Build history of the part. All positions in model axes, mm. A direction names the side the tool comes from. Give positions to 0.01 mm unless a question says otherwise; leave off trailing zeros. Order: outer loops, then holes, each group sorted by start corner. A loop starts at its lowest first (then second) coordinate and runs counter-clockwise, first axis right, second up. Notation, with made-up numbers: (-29, 32.5) - (-15, 32.5) arc R23 cw to (-15, 44.5) - close; hole circle Ø5 at (55.25, -6). An arc over 180 degrees is marked (long way). Use a Markdown table: item, result.
from build123d import *

# Parameters (mm, degrees)
CUT_EXTRUDE1_DEPTH      = 1.2
CUT_EXTRUDE1_DEPTH_BACK = 1.2


with BuildPart() as part:
    # Sketch1 → Revolve1 (revolve)
    with BuildSketch(Plane.XY):
        with BuildLine():
            Line((-1.782329983, 2.8), (0, 2.8))
            Line((0, 2.8), (0, 1.44675))
            ThreePointArc((0, 1.44675), (0.029289322, 1.376039322), (0.1, 1.34675))
            Line((0.1, 1.34675), (0.428063214, 1.34675))
            Line((0.428063214, 1.34675), (1, 1.5))
            Line((1, 1.5), (8, 1.5))
            Line((8, 1.5), (10, 1.218918331))
            Line((10, 1.218918331), (10, 0))
            Line((10, 0), (-2.4, 0))
            ThreePointArc((-2.4, 0), (-2.267625669, 1.393419223), (-1.875238613, 2.736986301))
            ThreePointArc((-1.875238613, 2.736986301), (-1.838460945, 2.782760589), (-1.782329983, 2.8))
        make_face()
    revolve(axis=Axis((13, 0, 0), (-1, 0, 0)))

    # Sketch2 → Cut-Extrude1 (cut, two sides)
    with BuildSketch(Plane(origin=(-2.4, 0, 0), x_dir=(0, 0, -1), z_dir=(1, 0, 0))) as cut_extrude1_sk:
        Polygon((-1.5, 0.375), (-1.5, -0.375), (-0.6, -0.296260203), (-0.375, -0.375), (-0.296260203, -0.6), (-0.375, -1.5), (0.375, -1.5), (0.296260203, -0.6), (0.375, -0.375), (0.6, -0.296260203), (1.5, -0.375), (1.5, 0.375), (0.6, 0.296260203), (0.375, 0.375), (0.296260203, 0.6), (0.375, 1.5), (-0.375, 1.5), (-0.296260203, 0.6), (-0.375, 0.375), (-0.6, 0.296260203), align=None)
    extrude(amount=CUT_EXTRUDE1_DEPTH, mode=Mode.SUBTRACT)
    extrude(cut_extrude1_sk.sketch, amount=-CUT_EXTRUDE1_DEPTH_BACK, mode=Mode.SUBTRACT)


solid = part.part
1) Wall check: line 1 (Z direction, x = 5.5, y = -0.1); line 2 (Z direction, x = 9, y = -0.2); line 3 (Z direction, x = -1.25, y = -1.3). Give the ranges that are in metal, low to high. Write a range as from..to.
Computed:
| item | result |
|---|---|
| line 1 | z = -1.5..1.5 |
| line 2 | z = -1.34..1.34 |
| line 3 | z = -2.48..-0.36, 0.36..2.48 |
2) Slice it at C-C (x = 3.5). Write the cut outline in (y, z).
Computed:
| item | result |
|---|---|
| outline | circle Ø3 at (0, 0) |
3) Slice it at D-D (x = -0.75). Write the cut outline in (y, z).
Computed:
| item | result |
|---|---|
| outline | circle Ø5.6 at (0, 0) |
4) Tool access for faces 5 (the cylindrical face through (-0.9, -2.8, -0.1)), 6 (the cylindrical face through (4.55, -1.5, -0.07)), 7 (the flat face through (-1.793, -0.336, 1.056)): list every direction of +Z, -Z, +X, -X, +Y, -Y with a clear straight run to the whole face (end or side of a thin tool).
Computed:
| item | result |
|---|---|
| face 5 | +X, -X |
| face 6 | +X |
| face 7 | -X |
5) Two-plate mould, pull along X, no slides. Class faces 1 (the flat face through (-1.2, 0, 0)), 2 (the flat face through (10, 0, 0)), 3 (the flat face through (-1.793, 0.335, 1.044)), 4 (the cylindrical face through (0.27, -1.07, 0.82)): +X half, -X half, draft (parallel to the pull), parting line (faces both ways), or undercut.
Computed:
| item | result |
|---|---|
| face 1 | -X half |
| face 2 | +X half |
| face 3 | draft |
| face 4 | undercut |
6) Pin check, flat tip, straight feed: P1, Ø2, axis at x = 3, y = -2, coming from the -Z side. Stop position of the tip, or through.
Computed:
| item | result |
|---|---|
| P1 | stops at z = -1.12 |
7) Slice it at A-A (y = 0). Write the cut outline in (x, z).
Computed:
| item | result |
|---|---|
| outline | (-2.25, -1.5) arc R7.4 ccw to (-1.88, -2.74) arc R0.1 ccw to (-1.78, -2.8) - (0, -2.8) - (0, -1.45) arc R0.1 cw to (0.1, -1.35) - (0.43, -1.35) - (1, -1.5) - (8, -1.5) - (10, -1.22) - (10, 1.22) - (8, 1.5) - (1, 1.5) - (0.43, 1.35) - (0.1, 1.35) arc R0.1 cw to (0, 1.45) - (0, 2.8) - (-1.78, 2.8) arc R0.1 ccw to (-1.88, 2.74) arc R7.4 ccw to (-2.25, 1.5) - (-1.2, 1.5) - (-1.2, -1.5) - close |
